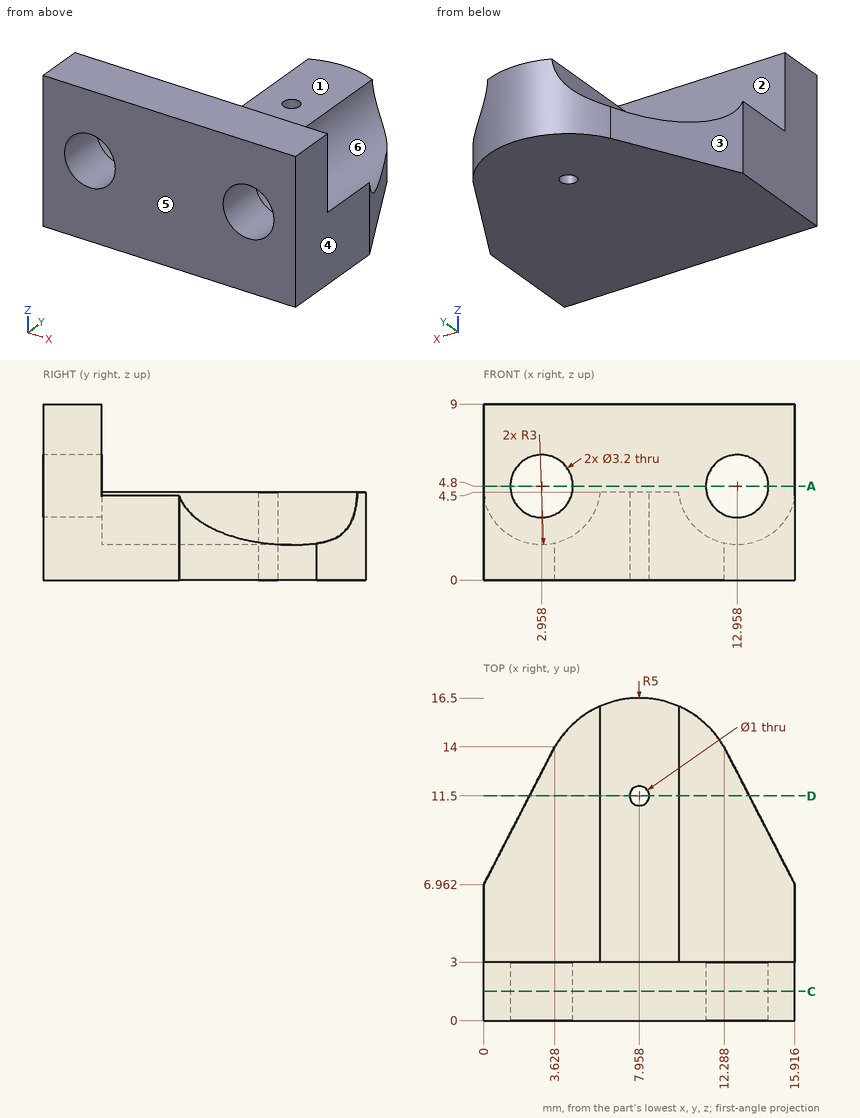
Input: dimensioned drawing with shaded views. Units: mm. Origin: part minimum x, y, z. A direction names the side the tool comes from. Coordinates: 2 decimals unless noted, no trailing zeros. Loops run counter-clockwise (first coordinate to the right, second up) from the corner with the lowest first, then second, coordinate; pieces in that order, holes last.
Q1. Section D-D, the plane y = 11.5. Return the cut outline in (x, z) (1 decimal), and give its area (3 significant figures).
Results are:
outline: (2.3, 0) - (7.5, 0) - (7.5, 4.5) - (5.9, 4.5) arc R3 cw to (2.3, 1.9) - close; (8.5, 0) - (13.6, 0) - (13.6, 1.9) arc R3 cw to (10, 4.5) - (8.5, 4.5) - close
area: 30.4 mm2
Q2. Line query: line 1 along Z through (x, y) = (13, 1.5); line 2 along X through (y, z) = (2.5, 4) (1 decimal); line 3 along Y through (x, z) = (12.75, 6.5). Output: solid intervals per line, ascending.
Results are:
line 1: z = 0 to 3.2, 6.4 to 9
line 2: x = 0 to 1.6, 4.3 to 11.6, 14.3 to 15.9
line 3: y = 0 to 3
Q3. Section A-A, the plane z = 4.8. Return the cut outline in (x, y).
Results are:
outline: (0, 0) - (1.36, 0) - (1.36, 3) - (0, 3) - close; (4.56, 0) - (11.36, 0) - (11.36, 3) - (4.56, 3) - close; (14.56, 0) - (15.92, 0) - (15.92, 3) - (14.56, 3) - close
Q4. Set-up query: the marked faces 5 and 6. Return all of +Z, -Z, +X, -X, +Y, -Y with unobstructed straight access to the full face (end or side cutting, diameter ignored); none if empty.
Results are:
face 5: +Z, -Z, +X, -X, -Y
face 6: +Z, +Y
Q5. Contact query for flat-ended pins moving along their axis: pin 1 (3 mm diameter, centred on x = 10.5, y = 9.5, fed in from +Z); pin 2 (3 mm diameter, centred on x = 2.958, z = 4.8, fed in from +Y); pin 3 (1 mm diameter, centred on x = 8, z = 7.5, fed in from +Y). Output: stop coordinate, or through.
Results are:
pin 1: stops at z = 4.5
pin 2: passes through
pin 3: stops at y = 3
Q6. Section C-C, the plane y = 1.5. Return the cut outline in (x, z), and give its area (3 significant figures).
Results are:
outline: (0, 0) - (15.92, 0) - (15.92, 9) - (0, 9) - close; hole circle Ø3.2 at (2.96, 4.8); hole circle Ø3.2 at (12.96, 4.8)
area: 127 mm2
Q7. Mould query, pull axis X, two halves, no side actions, for the marked faces 1, 2, 3 and 4. Classes: +X half, -X half, draft (parallel to the pull), parting line (faces both ways), or undercut.
Results are:
face 1: draft
face 2: undercut
face 3: -X half
face 4: +X half
